from build123d import *

# Parameters (mm, degrees)
BOSS_EXTRUDE1_DEPTH = 125
FILLET1_R           = 4
SKETCH2_R           = 2.5
CUT_EXTRUDE1_DEPTH  = 125


with BuildPart() as part:
    # Sketch1 → Boss-Extrude1 (new body)
    with BuildSketch(Plane(origin=(0, 0, 0), x_dir=(0, 0, -1), z_dir=(1, 0, 0))):
        Polygon((1.141646312, 16.786775831), (17.141646312, 16.786775831), (17.141646312, 18.786775831), (-0.858353688, 18.786775831), (-0.858353688, -16.213224169), (1.141646312, -16.213224169), align=None)
    extrude(amount=BOSS_EXTRUDE1_DEPTH)

    # Fillet1
    fillet1_edges = [part.edges().sort_by_distance(p)[0] for p in [
        (62.5, 18.786775831, 0.858353688),
    ]]
    fillet(fillet1_edges, radius=FILLET1_R)

    # Sketch2 → Cut-Extrude1 (cut)
    with BuildSketch(Plane(origin=(0, 0, -1.141646312), x_dir=(-1, 0, 0), z_dir=(0, 0, -1))):
        with Locations((-110, -11.213224169)):
            Circle(SKETCH2_R)
        with Locations((-15, -11.213224169)):
            Circle(SKETCH2_R)
    extrude(amount=-CUT_EXTRUDE1_DEPTH, mode=Mode.SUBTRACT)


solid = part.part
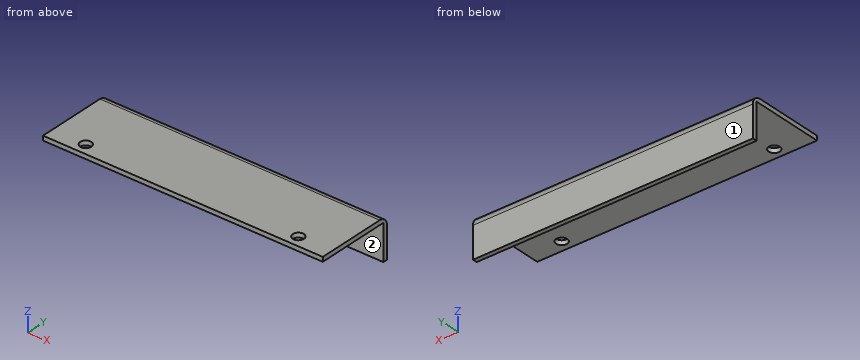
Geometry: final body of the model. Coordinates: model frame, mm. Face numbers are marked on the shaded views. A direction names the side the tool comes from. Give positions to 0.01 mm unless a question says otherwise; leave off trailing zeros. Loops run counter-clockwise (first coordinate to the right, second up) from the corner with the lowest first, then second, coordinate; pieces in that order, holes last. Notation, with made-up numbers: M 0,37 L 43,37 A8 ccw 43,43 Z; hole C -31,-39 d1. An arc over 180 degrees is marked long. Put each result on its own line as item: value.
1) Reachability of the marked faces 1 and 2 from +Z, -Z, +X, -X, +Y, -Y: full face, straight path, thin tool, end or side. Return the list, or none.
Computed values:
face 1: +Z, -Z, +X, -X, +Y
face 2: -Z, +X, -X, -Y
2) Cut plane C-C, the plane z = -12. Return the cut outline in (x, y), plus the area to 3 significant figures.
Computed values:
outline: M 0,16.79 L 125,16.79 L 125,18.79 L 0,18.79 Z
area: 250 mm^2
3) Cut plane A-A, the plane x = 110. Return the cut outline in (y, z), plus the area to 3 significant figures.
Computed values:
outline: M -16.21,-1.14 L -13.71,-1.14 L -13.71,0.86 L -16.21,0.86 Z; M -8.71,-1.14 L 16.79,-1.14 L 16.79,-17.14 L 18.79,-17.14 L 18.79,-3.14 A4 ccw 14.79,0.86 L -8.71,0.86 Z
area: 88.6 mm^2
4) Material intervals for L1, parallel to Z at x = 8.5, y = 3.5; L2, parallel to Y at x = 97, z = -3.5; L3, parallel to Y at x = 110, z = 0.4, sorted ascending. Write a range as from..to.
Computed values:
L1: z = -1.14..0.86
L2: y = 16.79..18.79
L3: y = -16.21..-13.71, -8.71..16.65
5) Cut plane B-B, the plane x = 31.5. Return the cut outline in (y, z).
Computed values:
outline: M -16.21,-1.14 L 16.79,-1.14 L 16.79,-17.14 L 18.79,-17.14 L 18.79,-3.14 A4 ccw 14.79,0.86 L -16.21,0.86 Z
6) First-contact query: P1, Ø3, axis at x = 49, z = -8, coming from the -Y side; P2, Ø16.5, axis at x = 87, y = -0.5, coming from the -Z side; P3, Ø4, axis at x = 110, y = -11.21, coming from the -Z side. Flat tips, straight axial feed; report the tip coordinate or a pass-through.
Computed values:
P1: stops at y = 16.79
P2: stops at z = -1.14
P3: passes through
7) Cut plane D-D, the plane y = 10. Return the cut outline in (x, z).
Computed values:
outline: M 0,-1.14 L 125,-1.14 L 125,0.86 L 0,0.86 Z
